Check sheet for the drawn part. Datum: minimum x, y, z corner. Units: mm. A direction names the side the tool comes from. Round coordinates to 2 decimals unless told otherwise and drop trailing zeros. Write each loop counter-clockwise with the first axis right and the second up, starting at its lowest first coordinate (ties: lowest second). Pieces come first, ordered by that corner, then holes. Notation, with made-up numbers: (88.5, -1.5) - (126.5, -1.5) arc R13 cw to (126.5, 13.5) - close; hole circle Ø4 at (36, 53.25). An arc over 180 degrees is marked (long way). Return JSON: item names as keys, results as strings. Group by question number.
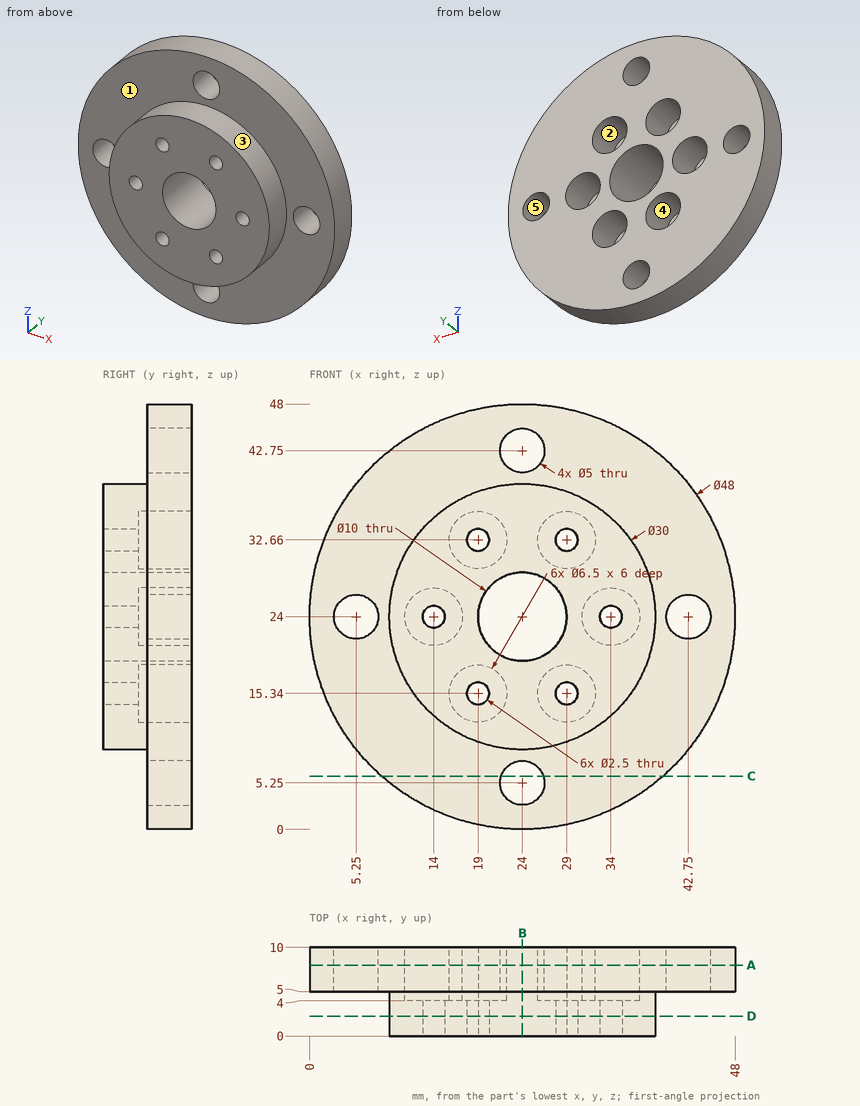
1. Section check B-B (x = 24). Enter the section's corners in (y, z).
2. Depth check by flat-ended pin: pin 1 Ø4 at (y, z) = (6.5, 30) entering from -X; pin 2 Ø5 at (x, y) = (36, 3.5) entering from +Z; pin 3 Ø5 at (x, z) = (14, 24) entering from +Y. Enter the tip coordinate at first touch or a pass-through.
3. Section check C-C (z = 6). Enter the section's corners in (x, y) (1 decimal), and give its area (3 significant figures).
4. Section check A-A (y = 8). State how many separate pieces and enclosed holes the cut face has, and give its area (3 significant figures).
5. Tool access check on the marked faces 4 and 5. Record the directions out of +Z, -Z, +X, -X, +Y, -Y that give a thin tool (end or side, any length) a straight path to the whole face; none if there is none.
6. Material ranges on line 1 along X through (y, z) = (2.1, 24); line 2 along X through (y, z) = (6.5, 24); line 3 along Z through (x, y) = (16.5, 4.25) (1 decimal), recorded low to high.
7. Mould release check, pull along X, two halves, no side actions. Record for the marked faces 1, 2 and 3: pulls with the +X half, pulls with the -X half, needs draft (parallel to the pull), parting line crosses it, or undercut.
8. Section check D-D (y = 2.25). Enter the section's corners in (x, z), and give its area (3 significant figures).
Result sheet:
{
 "1": {"outline": "(0, 9) - (5, 9) - (5, 7.75) - (10, 7.75) - (10, 19) - (0, 19) - close; (0, 29) - (10, 29) - (10, 40.25) - (5, 40.25) - (5, 39) - (0, 39) - close; (5, 0) - (10, 0) - (10, 2.75) - (5, 2.75) - close; (5, 45.25) - (10, 45.25) - (10, 48) - (5, 48) - close"},
 "2": {"pin 1": "stops at x = 0.34", "pin 2": "stops at z = 45.82", "pin 3": "stops at y = 4"},
 "3": {"outline": "(8.1, 5) - (21.6, 5) - (21.6, 10) - (8.1, 10) - close; (26.4, 5) - (39.9, 5) - (39.9, 10) - (26.4, 10) - close", "area": "135 mm²"},
 "4": {"separate pieces": "1", "enclosed holes": "11", "area": "1,450 mm²"},
 "5": {"face 4": "+Y", "face 5": "+Y, -Y"},
 "6": {"line 1": "x = 9 to 12.75, 15.25 to 19, 29 to 32.75, 35.25 to 39", "line 2": "x = 0 to 2.75, 7.75 to 10.75, 17.25 to 19, 29 to 30.75, 37.25 to 40.25, 45.25 to 48", "line 3": "z = 11 to 13.3, 17.4 to 21.9, 26.1 to 30.6, 34.7 to 37"},
 "7": {"face 1": "needs draft", "face 2": "undercut", "face 3": "parting line crosses it"},
 "8": {"outline": "circle Ø30 at (24, 24); hole circle Ø2.5 at (14, 24); hole circle Ø2.5 at (19, 15.34); hole circle Ø2.5 at (19, 32.66); hole circle Ø10 at (24, 24); hole circle Ø2.5 at (29, 15.34); hole circle Ø2.5 at (29, 32.66); hole circle Ø2.5 at (34, 24)", "area": "599 mm²"}
}
